from build123d import *

# Parameters (mm, degrees)
SKETCH1_R           = 3.96875
BOSS_EXTRUDE1_DEPTH = 6.35
SKETCH2_W           = 153.277121284
SKETCH2_H           = 15.875
SKETCH2_R           = 3.96875
BOSS_EXTRUDE2_DEPTH = 6.35
FILLET1_R           = 2.54
CUT_EXTRUDE1_DEPTH  = 16.875


with BuildPart() as part:
    # Sketch1 → Boss-Extrude1 (new body)
    with BuildSketch(Plane.XY):
        Polygon((0, 0), (0, 66.04), (95.25, 66.04), (153.277121284, 0), align=None)
        with Locations((9.525, 56.515)):
            Circle(SKETCH1_R, mode=Mode.SUBTRACT)
        with Locations((47.625, 56.515)):
            Circle(SKETCH1_R, mode=Mode.SUBTRACT)
        with Locations((85.725, 56.515)):
            Circle(SKETCH1_R, mode=Mode.SUBTRACT)
        Polygon((9.525, 14.756535386), (9.525, 46.99), (82.829969346, 46.99), align=None, mode=Mode.SUBTRACT)
        Polygon((21.290817509, 9.525), (101.311219354, 44.71135659), (132.228284487, 9.525), align=None, mode=Mode.SUBTRACT)
    extrude(amount=BOSS_EXTRUDE1_DEPTH)

    # Sketch2 → Boss-Extrude2 (add)
    with BuildSketch(Plane.XZ):
        with Locations((76.638560642, -7.9375)):
            Rectangle(SKETCH2_W, SKETCH2_H)
        with Locations((25.4, -9.525)):
            Circle(SKETCH2_R, mode=Mode.SUBTRACT)
        with Locations((76.2, -9.525)):
            Circle(SKETCH2_R, mode=Mode.SUBTRACT)
        with Locations((127, -9.525)):
            Circle(SKETCH2_R, mode=Mode.SUBTRACT)
    extrude(amount=-BOSS_EXTRUDE2_DEPTH)

    # Fillet1
    fillet1_edges = [part.edges().sort_by_distance(p)[0] for p in [
        (73.848795196, 6.35, 0),
    ]]
    fillet(fillet1_edges, radius=FILLET1_R)

    # Sketch3 → Cut-Extrude1 (cut, through all)
    with BuildSketch(Plane(origin=(0, 0, 0), x_dir=(-1, 0, 0), z_dir=(0, 0, -1))):
        Polygon((-153.277121284, 0), (-143.888240191, 10.685377693), (-163.562021825, 13.552350256), (-165.283233358, 4.245452075), align=None)
    extrude(amount=CUT_EXTRUDE1_DEPTH, mode=Mode.SUBTRACT)


solid = part.part
Input: part model. Units: mm. Frame: model coordinates. A direction names the side the tool comes from. Coordinates: 2 decimals unless noted, no trailing zeros. Loops run counter-clockwise (first coordinate to the right, second up) from the corner with the lowest first, then second, coordinate; pieces in that order, holes last. Notation, with made-up numbers: (75, 6.5) -> (123, 6.5) arc R21 cw to (123, 11.5) -> close; hole circle Ø7 at (-20.75, 88.5). An arc over 180 degrees is marked (long way). Write item = value, one per line. Start each with the question number.
Item 1: Cut plane C-C, the plane y = 12. Return loops of the section in (x, z), plus the area to 3 significant figures.
Item 2: Material intervals for line 1 (Y direction, x = 63, z = 4.25) (3 decimals); line 2 (Z direction, x = 127, y = 5) (3 decimals); line 3 (Y direction, x = 45.5, z = 2.25) (3 decimals), sorted ascending.
Item 3: Mould query, pull axis Z, two halves, no side actions, for faces 1 (the face through (74.883, 7.114, -0.724)), 2 (the face through (21.435, 3.131, -9.351)), 3 (the face through (130.666, 3.131, -11.045)), 4 (the face through (82.576, 54.1, 3.131)). Classes: pulls with the +Z half, pulls with the -Z half, needs draft (parallel to the pull), parting line crosses it, or undercut.
Item 4: Cut plane B-B, the plane x = 112. Return loops of the section in (y, z) (3 decimals).
Item 5: Reachability of faces 5 (the face through (58, 51, 0)), 6 (the face through (60.74, 26.87, 3.13)), 7 (the face through (76, 0, -5)) from +Z, -Z, +X, -X, +Y, -Y: full face, straight path, thin tool, end or side. Return the list, or none.
Item 6: Cut plane D-D, the plane y = 35. Return loops of the section in (x, z) (3 decimals), plus the area to 3 significant figures.
Item 7: First-contact query: P1, Ø7, axis at x = 85.725, y = 56.515, coming from the +Z side; P2, Ø2, axis at x = 117, y = 8, coming from the -Z side; P3, Ø10.5, axis at x = 76.2, z = -9.525, coming from the +Y side; P4, Ø2, axis at x = 39, y = 26.5, coming from the -Z side. Flat tips, straight axial feed; report the tip coordinate or a pass-through.
Item 8: Cut plane A-A, the plane y = 59. Return loops of the section in (x, z).
Ans:
q1.outline = (0, 0) -> (26.92, 0) -> (26.92, 6.35) -> (0, 6.35) -> close; (130.05, 0) -> (142.73, 0) -> (142.73, 6.35) -> (130.05, 6.35) -> close
q1.area = 251 mm²
q2.line_1 = 0 to 9.525, 27.865 to 38.27, 46.99 to 66.04
q2.line_2 = -15.875 to -13.494, -5.556 to 6.35
q2.line_3 = 0 to 9.525, 20.17 to 30.575, 46.99 to 53.163, 59.867 to 66.04
q3.face_1 = pulls with the -Z half
q3.face_2 = undercut
q3.face_3 = undercut
q3.face_4 = needs draft
q4.outline = (0, -15.875) -> (6.35, -15.875) -> (6.35, -2.54) arc R2.54 cw to (8.89, 0) -> (9.525, 0) -> (9.525, 6.35) -> (0, 6.35) -> close; (32.547, 0) -> (46.977, 0) -> (46.977, 6.35) -> (32.547, 6.35) -> close
q5.face_5 = -Z, +X, -X, +Y
q5.face_6 = +Z, -Z
q5.face_7 = +Z, -Z, +X, -X, -Y
q6.outline = (0, 0) -> (9.525, 0) -> (9.525, 6.35) -> (0, 6.35) -> close; (55.562, 0) -> (79.226, 0) -> (79.226, 6.35) -> (55.562, 6.35) -> close; (109.844, 0) -> (122.524, 0) -> (122.524, 6.35) -> (109.844, 6.35) -> close
q6.area = 291 mm²
q7.P1 = through
q7.P2 = -0.84
q7.P3 = 6.35
q7.P4 = 0
q8.outline = (0, 0) -> (6.43, 0) -> (6.43, 6.35) -> (0, 6.35) -> close; (12.62, 0) -> (44.53, 0) -> (44.53, 6.35) -> (12.62, 6.35) -> close; (50.72, 0) -> (82.63, 0) -> (82.63, 6.35) -> (50.72, 6.35) -> close; (88.82, 0) -> (101.44, 0) -> (101.44, 6.35) -> (88.82, 6.35) -> close
